Could you check a few things on this model? Use its own coordinates, in mm. A direction names the side the tool comes from. Round coordinates to 2 decimals unless told otherwise and drop trailing zeros. Loops run counter-clockwise (first coordinate to the right, second up) from the corner with the lowest first, then second, coordinate; pieces in that order, holes last.
from build123d import *

# Parameters (mm, degrees)
BOSS_EXTRUDE1_DEPTH                     = 25
BOSS_EXTRUDE2_START                     = -25
BOSS_EXTRUDE2_DEPTH                     = 35
CBORE_FOR_M8_HEX_HEAD_BOLT2_D           = 8.4
CBORE_FOR_M8_HEX_HEAD_BOLT2_CBORE_D     = 18.01
CBORE_FOR_M8_HEX_HEAD_BOLT2_CBORE_DEPTH = 5.68
CUT_EXTRUDE1_DEPTH                      = 20
BOSS_EXTRUDE3_START                     = -25
BOSS_EXTRUDE3_DEPTH                     = 95
SKETCH10_R                              = 38.33
SKETCH10_R_2                            = 20.5
BOSS_EXTRUDE4_DEPTH                     = 120
CUT_EXTRUDE2_DEPTH                      = 130
SKETCH12_R                              = 38.33
SKETCH12_R_2                            = 20.5
BOSS_EXTRUDE5_DEPTH                     = 120
CUT_EXTRUDE3_DEPTH                      = 130
BOSS_EXTRUDE6_START                     = 10
SKETCH10_2_R                            = 38.33
SKETCH10_2_R_2                          = 20.5
BOSS_EXTRUDE6_DEPTH                     = 10
BOSS_EXTRUDE7_START                     = 10
SKETCH12_3_R                            = 38.33
SKETCH12_3_R_2                          = 20.5
BOSS_EXTRUDE7_DEPTH                     = 10
CHAMFER1_SIZE                           = 2


with BuildPart() as part:
    # Sketch1 → Boss-Extrude1 (new body)
    with BuildSketch(Plane(origin=(0, 0, 0), x_dir=(1, 0, 0), z_dir=(0, 1, 0))):
        with BuildLine():
            Line((10, 0), (190, 0))
            ThreePointArc((190, 0), (197.071067812, 2.928932188), (200, 10))
            Line((200, 10), (200, 203))
            ThreePointArc((200, 203), (197.071067812, 210.071067812), (190, 213))
            Line((190, 213), (10, 213))
            ThreePointArc((10, 213), (2.928932188, 210.071067812), (0, 203))
            Line((0, 203), (0, 10))
            ThreePointArc((0, 10), (2.928932188, 2.928932188), (10, 0))
        make_face()
    extrude(amount=BOSS_EXTRUDE1_DEPTH)

    # Sketch2 → Boss-Extrude2 (add)
    with BuildSketch(Plane(origin=(0, 25, 0), x_dir=(1, 0, 0), z_dir=(0, 1, 0)).offset(BOSS_EXTRUDE2_START)):
        with BuildLine():
            Line((155, 60), (200, 60))
            Line((200, 60), (200, 10))
            ThreePointArc((200, 10), (197.071067812, 2.928932188), (190, 0))
            Line((190, 0), (140, 0))
            Line((140, 0), (140, 45))
            ThreePointArc((140, 45), (144.393398282, 55.606601718), (155, 60))
        make_face()
    extrude(amount=BOSS_EXTRUDE2_DEPTH)

    # CBORE for M8 Hex Head Bolt2 (through all)
    with Locations(Plane(origin=(170, 35, -30), x_dir=(0, 0, 1), z_dir=(0, 1, 0))):
        with Locations((0, 0)):
            CounterBoreHole(CBORE_FOR_M8_HEX_HEAD_BOLT2_D / 2, CBORE_FOR_M8_HEX_HEAD_BOLT2_CBORE_D / 2, CBORE_FOR_M8_HEX_HEAD_BOLT2_CBORE_DEPTH)

    # Sketch9 → Cut-Extrude1 (cut)
    with BuildSketch(Plane(origin=(0, 25, 0), x_dir=(1, 0, 0), z_dir=(0, 1, 0))):
        with BuildLine():
            ThreePointArc((54, 51.509494051), (55.833002466, 56.953219461), (60.585365854, 60.179531072))
            ThreePointArc((60.585365854, 60.179531072), (110.610173055, 89.389826945), (139.820468928, 139.414634146))
            ThreePointArc((139.820468928, 139.414634146), (143.046780539, 144.166997534), (148.490505949, 146))
            Line((148.490505949, 146), (182, 146))
            ThreePointArc((182, 146), (188.363961031, 143.363961031), (191, 137))
            Line((191, 137), (191, 78))
            ThreePointArc((191, 78), (188.363961031, 71.636038969), (182, 69))
            Line((182, 69), (140, 69))
            ThreePointArc((140, 69), (133.636038969, 66.363961031), (131, 60))
            Line((131, 60), (131, 18))
            ThreePointArc((131, 18), (128.363961031, 11.636038969), (122, 9))
            Line((122, 9), (63, 9))
            ThreePointArc((63, 9), (56.636038969, 11.636038969), (54, 18))
            Line((54, 18), (54, 51.509494051))
        make_face()
    extrude(amount=-CUT_EXTRUDE1_DEPTH, mode=Mode.SUBTRACT)

    # Sketch9<3> → Boss-Extrude3 (add)
    with BuildSketch(Plane(origin=(0, 25, 0), x_dir=(1, 0, 0), z_dir=(0, 1, 0)).offset(BOSS_EXTRUDE3_START)):
        with BuildLine():
            Line((200, 155), (200, 170))
            Line((200, 170), (120, 170))
            ThreePointArc((120, 170), (93.639610307, 106.360389693), (30, 80))
            Line((30, 80), (30, 0))
            Line((30, 0), (45, 0))
            Line((45, 0), (45, 66.076951546))
            ThreePointArc((45, 66.076951546), (104.246212025, 95.753787975), (133.923048454, 155))
            Line((133.923048454, 155), (200, 155))
        make_face()
    extrude(amount=BOSS_EXTRUDE3_DEPTH)

    # Sketch10 → Boss-Extrude4 (add)
    with BuildSketch(Plane(origin=(200, 0, 0), x_dir=(0, 0, -1), z_dir=(1, 0, 0))):
        with Locations((162.5, 95)):
            Circle(SKETCH10_R)
        with Locations((162.5, 95)):
            Circle(SKETCH10_R_2, mode=Mode.SUBTRACT)
    extrude(amount=-BOSS_EXTRUDE4_DEPTH)

    # Sketch11 → Cut-Extrude2 (cut)
    with BuildSketch(Plane(origin=(200, 0, 0), x_dir=(0, 0, -1), z_dir=(1, 0, 0))):
        with BuildLine():
            Line((142, 95), (170, 95))
            Line((170, 95), (170, 75.921215972))
            ThreePointArc((170, 75.921215972), (150.956603619, 78.058925654), (142, 95))
        make_face()
    extrude(amount=-CUT_EXTRUDE2_DEPTH, mode=Mode.SUBTRACT)

    # Sketch12 → Boss-Extrude5 (add)
    with BuildSketch(Plane.XY):
        with Locations((37.5, 95)):
            Circle(SKETCH12_R)
        with Locations((37.5, 95)):
            Circle(SKETCH12_R_2, mode=Mode.SUBTRACT)
    extrude(amount=-BOSS_EXTRUDE5_DEPTH)

    # Sketch13 → Cut-Extrude3 (cut)
    with BuildSketch(Plane.XY):
        with BuildLine():
            Line((25.688032589, 78.245077563), (25.688032589, 100.102181985))
            Line((25.688032589, 100.102181985), (51.572180065, 100.102181985))
            Line((51.572180065, 100.102181985), (58, 95))
            ThreePointArc((58, 95), (46.936754423, 76.80116306), (25.688032589, 78.245077563))
        make_face()
    extrude(amount=-CUT_EXTRUDE3_DEPTH, mode=Mode.SUBTRACT)

    # Sketch10<2> → Boss-Extrude6 (add)
    with BuildSketch(Plane(origin=(200, 0, 0), x_dir=(0, 0, -1), z_dir=(1, 0, 0)).offset(BOSS_EXTRUDE6_START)):
        with Locations((162.5, 95)):
            Circle(SKETCH10_2_R)
        with Locations((162.5, 95)):
            Circle(SKETCH10_2_R_2, mode=Mode.SUBTRACT)
    extrude(amount=-BOSS_EXTRUDE6_DEPTH)

    # Sketch12<3> → Boss-Extrude7 (add)
    with BuildSketch(Plane.XY.offset(BOSS_EXTRUDE7_START)):
        with Locations((37.5, 95)):
            Circle(SKETCH12_3_R)
        with Locations((37.5, 95)):
            Circle(SKETCH12_3_R_2, mode=Mode.SUBTRACT)
    extrude(amount=-BOSS_EXTRUDE7_DEPTH)

    # Chamfer1
    chamfer1_edges = [part.edges().sort_by_distance(p)[0] for p in [
        (80, 95, -142),
        (17, 95, -120),
        (210, 95, -142),
        (17, 95, 10),
    ]]
    chamfer(chamfer1_edges, length=CHAMFER1_SIZE)


solid = part.part
Item 1: We'd pull the mould along Z, two halves only. Please class faces 5 (the flat face through (101, 12, -213)), 6 (the flat face through (123, 5, -78)), 7 (the flat face through (0, 12, -108)): released by +Z, released by -Z, zero draft, split by the parting line, or undercut.
Results list:
face 5: released by -Z
face 6: undercut
face 7: zero draft
Item 2: For faces 1 (the flat face through (54, 79, -120)), 2 (the cylindrical face through (55.784, 15.14, -56.888)), 3 (the cylindrical face through (2.85, 12.32, -3.01)), 4 (the flat face through (30, 41, -41)), which set-ups out of +Z, -Z, +X, -X, +Y, -Y let a thin tool reach every point of the face, with its end or its side?
Results list:
face 1: -Z, -X, +Y
face 2: none
face 3: +Z, -X, -Y
face 4: +Z, -Z, -X
Item 3: If I drill on line 1 along X through (y, z) = (33.4, -30) (3 decimals); line 2 along X through (y, z) = (10.5, -30); line 3 along Y through (x, z) = (127, -162), over which ranges is the centre line in solid material (lowest first)?
Results list:
line 1: x = 30 to 45, 140 to 160.995, 179.005 to 200
line 2: x = 0 to 54, 131 to 165.8, 174.2 to 200
line 3: y = 0 to 74.51, 115.49 to 133.33
Item 4: If we section it at B-B, the plane z = -95.5: Please give me the cut outline in (x, y), then the cut area to 3 significant figures.
Results list:
outline: circle Ø76.66 at (37.5, 95); (0, 0) - (200, 0) - (200, 25) - (191, 25) - (191, 5) - (116.29, 5) - (116.29, 25) - (103.99, 25) - (103.99, 95) - (80.5, 95) - (80.5, 25) - (0, 25) - close; hole circle Ø41 at (37.5, 95)
area: 8,450 mm2
Item 5: If we section it at D-D, the plane z = -162.5: Please give me the cut outline in (x, y).
Results list:
outline: (0, 0) - (200, 0) - (200, 56.67) - (210, 56.67) - (210, 72.5) - (208, 74.5) - (82, 74.5) - (80, 72.5) - (80, 56.67) - (119.69, 56.67) - (119.69, 25) - (0, 25) - close; (80, 117.5) - (82, 115.5) - (208, 115.5) - (210, 117.5) - (210, 133.33) - (80, 133.33) - close
Item 6: If we section it at A-A, the plane x = 170: Please give me the cut outline in (y, z) (3 decimals).
Results list:
outline: (0, -213) - (25, -213) - (25, -170) - (57.411, -170) arc R38.33 ccw (long way) to (57.411, -155) - (25, -155) - (25, -146) - (5, -146) - (5, -69) - (25, -69) - (25, -60) - (35, -60) - (35, -39.005) - (29.32, -39.005) - (29.32, -34.2) - (0, -34.2) - close; (0, -25.8) - (29.32, -25.8) - (29.32, -20.995) - (35, -20.995) - (35, 0) - (0, 0) - close; hole circle Ø41 at (95, -162.5)
Item 7: If we section it at C-C, the plane x = 37.5: Please give me the cut outline in (y, z).
Results list:
outline: (0, -213) - (25, -213) - (25, -80.31) - (56.67, -80.31) - (56.67, -120) - (72.5, -120) - (74.5, -118) - (74.5, 8) - (72.5, 10) - (56.67, 10) - (56.67, 0) - (0, 0) - close; (115.5, -118) - (117.5, -120) - (133.33, -120) - (133.33, 10) - (117.5, 10) - (115.5, 8) - close
Item 8: Will these pins go through, and if not, where does the flat tip stop? pin 1 (5 mm diameter, centred on x = 181.5, y = 28, fed in from +Z); pin 2 (6 mm diameter, centred on x = 139, y = 81, fed in from -Z); pin 3 (5 mm diameter, centred on x = 172, y = 32.5, fed in from -Z).
Results list:
pin 1: stops at z = 0
pin 2: stops at z = -199.22
pin 3: stops at z = -170
